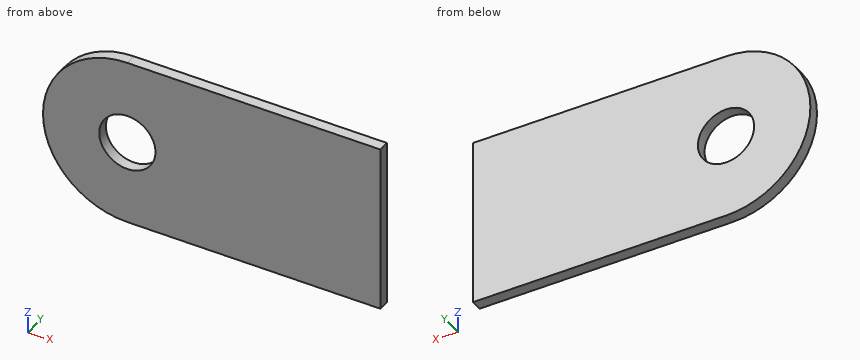
from build123d import *

# Parameters (mm, degrees)
F0_R     = 5
F1_DEPTH = 2


with BuildPart() as f1:
    # F0 (on Front) → F1 (new body)
    with BuildSketch(Plane.XZ):
        with BuildLine():
            Line((0, -30), (0, 0))
            Line((0, 0), (-45, 0))
            ThreePointArc((-45, 0), (-55.606602, -4.393398), (-60, -15))
            ThreePointArc((-60, -15), (-55.606602, -25.606602), (-45, -30))
            Line((-45, -30), (0, -30))
        make_face()
        with Locations((-45, -15)):
            Circle(F0_R, mode=Mode.SUBTRACT)
    extrude(amount=F1_DEPTH)


solid = f1.part
Model file for the job. Use its own axes, mm. Round coordinates to 2 decimals unless told otherwise and drop trailing zeros. Loops run counter-clockwise (first coordinate to the right, second up) from the corner with the lowest first, then second, coordinate; pieces in that order, holes last. Notation, with made-up numbers: (32, 46.5) - (84, 46.5) arc R19 cw to (84, 82.5) - close; hole circle Ø10 at (71.25, 45.5). An arc over 180 degrees is marked (long way). Write each question's results on one line, items separated by ' | '.
(1) Wall check: L1, parallel to Z at x = -45, y = -0.7; L2, parallel to X at y = -0.6, z = -12.5; L3, parallel to X at y = -1.6, z = -12. Give the ranges that are in metal, low to high.
Answer below:
L1: z = -30 to -20, -10 to 0 | L2: x = -59.79 to -49.33, -40.67 to 0 | L3: x = -59.7 to -49, -41 to 0
(2) Saw through at B-B, the plane z = -24. List the corners of the cut face in (x, y), then the cut area to 3 significant figures.
Answer below:
outline: (-57, -2) - (0, -2) - (0, 0) - (-57, 0) - close | area: 114 mm^2
(3) Saw through at C-C, the plane x = -51. List the corners of the cut face in (y, z).
Answer below:
outline: (-2, -28.75) - (0, -28.75) - (0, -1.25) - (-2, -1.25) - close
(4) Saw through at A-A, the plane y = -1.05. List the corners of the cut face in (x, z), then the cut area to 3 significant figures.
Answer below:
outline: (-60, -15) arc R15 ccw to (-45, -30) - (0, -30) - (0, 0) - (-45, 0) arc R15 ccw to start; hole circle Ø10 at (-45, -15) | area: 1,620 mm^2
